CAD build for the part. Positions are in the model's coordinates, mm. Face numbers are marked on the shaded views. A direction names the side the tool comes from. Coordinates: 2 decimals unless noted, no trailing zeros. Loops run counter-clockwise (first coordinate to the right, second up) from the corner with the lowest first, then second, coordinate; pieces in that order, holes last. Notation, with made-up numbers: (32.5, 48.5) - (77.5, 48.5) arc R15 ccw to (77.5, 59.5) - close; hole circle Ø5 at (21, -36.75). An arc over 180 degrees is marked (long way). Put each result on its own line as item: value.
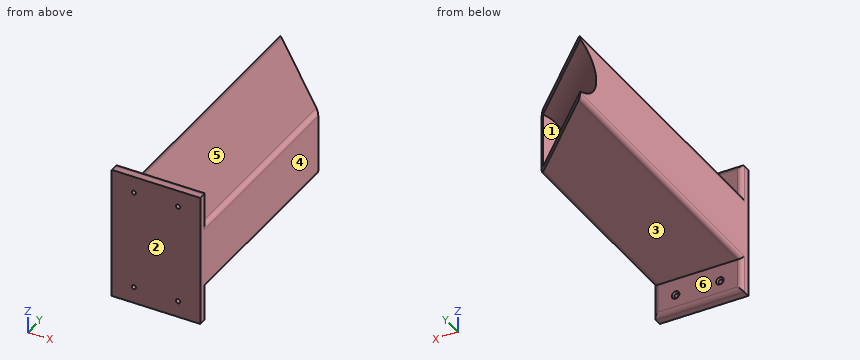
```python
from build123d import *

# Parameters (mm, degrees)
SKETCH1_W                                         = 50.8
SKETCH1_H                                         = 76.2
BOSS_EXTRUDE1_DEPTH                               = 6.35
SKETCH2_W                                         = 50.8
SKETCH2_H                                         = 38.1
BOSS_EXTRUDE2_DEPTH                               = 171.6066
CUT_EXTRUDE1_DEPTH                                = 183.535025619
CUT_EXTRUDE1_DEPTH_BACK                           = 183.535025619
BOSS_EXTRUDE3_REACH                               = 237.296
SKETCH20_W                                        = 38.1
SKETCH20_H                                        = 2.54
BOSS_EXTRUDE4_REACH                               = 129.523
CSK_FOR_2_FLAT_HEAD_MACHINE_SCREW_100_D           = 2.4384
CSK_FOR_2_FLAT_HEAD_MACHINE_SCREW_100_CSINK_D     = 4.3688
CSK_FOR_2_FLAT_HEAD_MACHINE_SCREW_100_CSINK_ANGLE = 100
FILLET1_R                                         = 2.54
FILLET2_R                                         = 2.54


with BuildPart() as part:
    # Sketch1 → Boss-Extrude1 (new body)
    with BuildSketch(Plane(origin=(0, 0, 0), x_dir=(1, 0, 0), z_dir=(0, 1, 0))):
        with Locations((-132.195454545, 0)):
            Rectangle(SKETCH1_W, SKETCH1_H)
    extrude(amount=BOSS_EXTRUDE1_DEPTH)

    # Sketch2 → Boss-Extrude2 (add)
    with BuildSketch(Plane(origin=(0, 6.35, 0), x_dir=(1, 0, 0), z_dir=(0, 1, 0))):
        with Locations((-132.195454545, 0)):
            Rectangle(SKETCH2_W, SKETCH2_H)
    extrude(amount=BOSS_EXTRUDE2_DEPTH)

    # Sketch19 → Cut-Extrude1 (cut, two sides: drawn at the far end of the back side and taken through both)
    with BuildSketch(Plane(origin=(-167.776027273, 167.776027273, 0), x_dir=(-0.7071067811865488, -0.7071067811865462, 0), z_dir=(0.7071067811865462, -0.7071067811865488, 0)).offset(-CUT_EXTRUDE1_DEPTH_BACK)):
        with BuildLine():
            Line((-14.397504024, 16.51), (-14.397504024, -16.51))
            ThreePointArc((-14.397504024, -16.51), (2.112495976, 0), (-14.397504024, 16.51))
        make_face()
    extrude(amount=CUT_EXTRUDE1_DEPTH + CUT_EXTRUDE1_DEPTH_BACK, mode=Mode.SUBTRACT)

    # SurfaceCut1
    split(bisect_by=Plane(origin=(6.588470279, 6.588470279, 0), x_dir=(0, 0, 1), z_dir=(-0.7071067811865488, -0.7071067811865464, 0)), keep=Keep.TOP)

    # Sketch20 → Boss-Extrude3 (add, up to next)
    with BuildSketch(Plane(origin=(6.588470279, 6.588470279, 0), x_dir=(0, 0, -1), z_dir=(0.7071067811865487, 0.7071067811865465, 0)), mode=Mode.PRIVATE) as boss_extrude3_sk1:
        with Locations((0, 161.619084242)):
            Rectangle(SKETCH20_W, SKETCH20_H)
    boss_extrude3_tool1 = extrude(boss_extrude3_sk1.sketch, amount=-BOSS_EXTRUDE3_REACH, mode=Mode.PRIVATE) - part.part
    add(boss_extrude3_tool1.solids().sort_by_distance((-107.69348, 120.870421, 0))[0])

    # Boss-Extrude4: up to this face of the body (flat: up to its plane)
    boss_extrude4_end = Plane(part.part.faces().sort_by_distance((-106.795454545, 52.426789341, 0))[0])
    # Sketch22 → Boss-Extrude4 (add, up to the picked face)
    with BuildSketch(Plane(origin=(-113.383924824, 113.383924824, 0), x_dir=(0, 0, -1), z_dir=(0.7071067811865465, -0.7071067811865486, 0)), mode=Mode.PRIVATE) as boss_extrude4_sk1:
        with BuildLine():
            Line((-15.709032434, 9.317504024), (15.709032434, 9.317504024))
            ThreePointArc((15.709032434, 9.317504024), (0, -6.39152841), (-15.709032434, 9.317504024))
        make_face()
    boss_extrude4_tool1 = split(extrude(boss_extrude4_sk1.sketch, amount=BOSS_EXTRUDE4_REACH, mode=Mode.PRIVATE), bisect_by=boss_extrude4_end, keep=Keep.BOTH, mode=Mode.PRIVATE)
    add(boss_extrude4_tool1.solids().sort_by(Axis((-111.509821, 115.258029, 0), (0.7071067811865465, -0.7071067811865486, 0)))[0])

    # CSK for #2 Flat Head Machine Screw (100)1 (through all)
    with Locations(Plane(origin=(0, 6.35, 0), x_dir=(1, 0, 0), z_dir=(0, 1, 0))):
        with Locations((-144.895454545, -28.575), (-119.495454545, -28.575)):
            csk_for_2_flat_head_machine_screw_100 = CounterSinkHole(CSK_FOR_2_FLAT_HEAD_MACHINE_SCREW_100_D / 2, CSK_FOR_2_FLAT_HEAD_MACHINE_SCREW_100_CSINK_D / 2, counter_sink_angle=CSK_FOR_2_FLAT_HEAD_MACHINE_SCREW_100_CSINK_ANGLE)

    # Mirror1: CSK for #2 Flat Head Machine Screw (100)1 across plane
    add(csk_for_2_flat_head_machine_screw_100.mirror(Plane.XY), mode=Mode.SUBTRACT)

    # Fillet1
    fillet1_edges = [part.edges().sort_by_distance(p)[0] for p in [
        (-157.595454545, 88.561197552, 19.05),
        (-106.795454545, 63.161197552, 19.05),
        (-106.795454545, 63.161197552, -19.05),
        (-157.595454545, 88.561197552, -19.05),
    ]]
    fillet(fillet1_edges, radius=FILLET1_R)

    # Fillet2
    fillet2_edges = [part.edges().sort_by_distance(p)[0] for p in [
        (-157.595454545, 6.35, -27.305),
        (-132.195454545, 6.35, -38.1),
        (-106.795454545, 6.35, -27.305),
        (-157.595454545, 6.35, 27.305),
        (-132.195454545, 6.35, 38.1),
        (-106.795454545, 6.35, 27.305),
    ]]
    fillet(fillet2_edges, radius=FILLET2_R)


solid = part.part
```
Q1. Slice it at B-B, the plane y = 30. Give the cut face in (x, z).
Determined:
outline: (-157.6, -16.51) arc R2.54 ccw to (-155.06, -19.05) - (-109.34, -19.05) arc R2.54 ccw to (-106.8, -16.51) - (-106.8, 16.51) arc R2.54 ccw to (-109.34, 19.05) - (-155.06, 19.05) arc R2.54 ccw to (-157.6, 16.51) - close
Q2. Slice it at A-A, the plane z = -24. Give the cut face in (x, y), then the cut area to 3 significant figures.
Determined:
outline: (-157.6, 0) - (-106.8, 0) - (-106.8, 3.81) arc R2.54 ccw to (-109.34, 6.35) - (-155.06, 6.35) arc R2.54 ccw to (-157.6, 3.81) - close
area: 320 mm2
Q3. Slice it at C-C, the plane z = 12.5. Give the cut face in (x, y).
Determined:
outline: (-157.6, 0) - (-106.8, 0) - (-106.8, 119.97) - (-108.59, 121.77) - (-112.63, 117.73) - (-157.6, 162.7) - close
Q4. Pin check, flat tips, straight feed: pin 1 Ø6 at (y, z) = (121, 19) entering from -X; pin 2 Ø3 at (x, z) = (-115, 5.5) entering from +Y; pin 3 Ø3 at (x, z) = (-144.9, 28.58) entering from +Y; pin 4 Ø5 at (x, z) = (-147, -10.5) entering from +Y. Stop position of each tip, or through.
Determined:
pin 1: x = -157.6
pin 2: y = 116.86
pin 3: y = 5.78
pin 4: y = 153.63
Q5. Wall check: L1, parallel to Z at x = -128, y = 138.5; L2, parallel to Z at x = -132, y = 32; L3, parallel to Y at x = -140.5, z = 25. Give the ranges that are in metal, low to high. Write a range as from..to.
Determined:
L1: -19.05..-14.97, 14.97..19.05
L2: -19.05..19.05
L3: 0..6.35
Q6. Tool access for the marked faces 4, 5 and 6: list every direction of +Z, -Z, +X, -X, +Y, -Y with a clear straight run to the whole face (end or side of a thin tool).
Determined:
face 4: +Z, -Z, +X, +Y, -Y
face 5: +Z, +X, -X, +Y
face 6: -Z, +X, -X, +Y
Q7. Mould opens along Z. For the marked faces 1, 2 and 3 say: +Z half, -Z half, draft (parallel to the pull), parting line (faces both ways), or undercut.
Determined:
face 1: undercut
face 2: draft
face 3: -Z half
